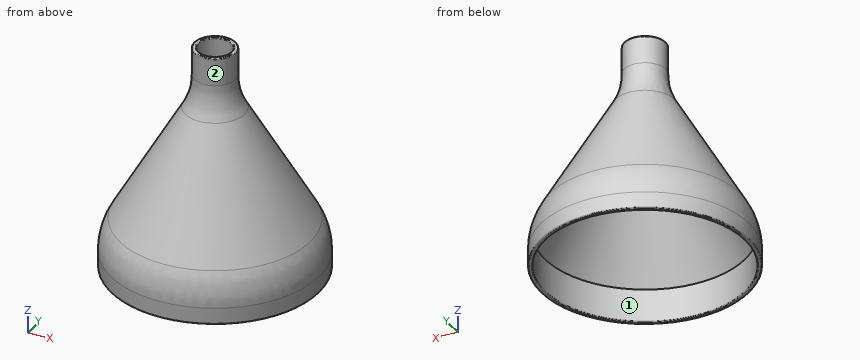
from build123d import *

# Parameters (mm, degrees)
F2_R = 20
F3_R = 0.3
F4_R = 0.3


with BuildPart() as f1:
    # F0 (on Front) → F1 (revolve)
    with BuildSketch(Plane.XZ):
        Polygon((-31.2, 0), (-30, 0), (-30, 10), (-5, 53.30127), (-5, 67.30127), (-6.2, 67.30127), (-6.2, 53.622809), (-31.2, 10.321539), align=None)
    revolve(axis=Axis((0, 0, 8.207551), (0, 0, 1)))

    # F2
    f2_edges = [f1.edges().sort_by_distance(p)[0] for p in [
        (31.2, 0, 10.321539),
        (6.2, 0, 53.622809),
    ]]
    fillet(f2_edges, radius=F2_R)

    # F3
    f3_edges = [f1.edges().sort_by_distance(p)[0] for p in [
        (5, 0, 67.30127),
        (6.2, 0, 67.30127),
    ]]
    fillet(f3_edges, radius=F3_R)

    # F4
    f4_edges = [f1.edges().sort_by_distance(p)[0] for p in [
        (31.2, 0, 0),
        (30, 0, 0),
    ]]
    fillet(f4_edges, radius=F4_R)


solid = f1.part
Check sheet for the modelled part. Datum: model origin and axes. Units: mm. Face numbers are marked on the shaded views. Round coordinates to 2 decimals unless told otherwise and drop trailing zeros. Write each loop counter-clockwise with the first axis right and the second up, starting at its lowest first coordinate (ties: lowest second). Pieces come first, ordered by that corner, then holes. Notation, with made-up numbers: (51.25, -16) -> (69.25, -16) arc R12 cw to (69.25, 0) -> close; hole circle Ø7 at (54, 59.25). An arc over 180 degrees is marked (long way). Answer as CSV lines item,"result". Start each with the question number.
1) Material ranges on line 1 (Y direction, x = 0, z = 62.25); line 2 (X direction, y = 0, z = 5.25), recorded low to high. Write a range as from..to.
2) Release check for a two-part mould opening along Y. For the marked faces 1 and 2 record: pulls with the +Y half, pulls with the -Y half, needs draft (parallel to the pull), parting line crosses it, or undercut.
3) Section check A-A on z = 24.5. Enter the section's corners in (x, y), and give its area (3 significant figures).
4) Go/stop test with flat-tipped pins: P1, Ø8, axis at y = 5, z = 52.5, coming from the +X side; P2, Ø11.5, axis at x = 0, y = 0, coming from the -Z side; P3, Ø2, axis at y = 5, z = 24, coming from the +X side. Record where each tip stops, or that it passes through.
Found:
1,line 1,"y = -6.2..-5, 5..6.2"
1,line 2,"x = -31.2..-30, 30..31.2"
2,face 1,"undercut"
2,face 2,"parting line crosses it"
3,outline,"circle Ø46.03 at (0, 0); hole circle Ø43.26 at (0, 0)"
3,area,"194 mm^2"
4,P1,"stops at x = 8.32"
4,P2,"stops at z = 52"
4,P3,"stops at x = 23.39"
